from build123d import *

# Parameters (mm, degrees)
BOSS_EXTRU_1_DEPTH      = 55
ESQUISSE2_W             = 35.5
ESQUISSE2_H             = 2
BOSS_EXTRU_2_DEPTH      = 1
BOSS_EXTRU_3_DEPTH      = 31.5
ESQUISSE4_W             = 8
ESQUISSE4_H             = 6.5
BOSS_EXTRU_4_DEPTH      = 2
ESQUISSE5_W             = 4.9
ESQUISSE5_H             = 1.9
BOSS_EXTRU_5_DEPTH      = 2
BOSS_EXTRU_6_DEPTH      = 3
ESQUISSE8_W             = 29.5
ESQUISSE8_H             = 49
ENL_V_MAT_EXTRU_2_DEPTH = 1
CONG_1_R                = 2
CONG_4_R                = 1.5
ESQUISSE7_R             = 6
ENL_V_MAT_EXTRU_1_DEPTH = 67.304223093


with BuildPart() as part:
    # Esquisse1 → Boss.-Extru.1 (new body)
    with BuildSketch(Plane.XY):
        Polygon((0, 0), (-2, 0), (-2, -1), (33.5, -1), (33.5, 0), (31.5, 0), (31.5, 2), (0, 2), align=None)
    extrude(amount=BOSS_EXTRU_1_DEPTH)

    # Esquisse2 → Boss.-Extru.2 (add)
    with BuildSketch(Plane.XZ.offset(1)):
        with Locations((15.75, 56)):
            Rectangle(ESQUISSE2_W, ESQUISSE2_H)
    extrude(amount=-BOSS_EXTRU_2_DEPTH)

    # Esquisse3 → Boss.-Extru.3 (add)
    with BuildSketch(Plane.ZY):
        Polygon((55, 2), (55, 2.1), (57, 2.1), (57, 4.1), (53, 4.1), (53, 2), align=None)
    extrude(amount=-BOSS_EXTRU_3_DEPTH)

    # Esquisse4 → Boss.-Extru.4 (add)
    with BuildSketch(Plane(origin=(0, 0, 0), x_dir=(-1, 0, 0), z_dir=(0, 0, -1))):
        with Locations((-15.75, 3.75)):
            Rectangle(ESQUISSE4_W, ESQUISSE4_H)
    extrude(amount=BOSS_EXTRU_4_DEPTH)

    # Esquisse5 → Boss.-Extru.5 (add)
    with BuildSketch(Plane.XY):
        with Locations((15.75, 5)):
            Rectangle(ESQUISSE5_W, ESQUISSE5_H)
    extrude(amount=BOSS_EXTRU_5_DEPTH)

    # Esquisse6 → Boss.-Extru.6 (add)
    with BuildSketch(Plane.XZ.offset(1)):
        with BuildLine():
            Line((5.75, 0), (5.75, -5))
            ThreePointArc((5.75, -5), (7.214466094, -8.535533906), (10.75, -10))
            Line((10.75, -10), (20.75, -10))
            ThreePointArc((20.75, -10), (24.285533906, -8.535533906), (25.75, -5))
            Line((25.75, -5), (25.75, 0))
            Line((25.75, 0), (5.75, 0))
        make_face()
    extrude(amount=-BOSS_EXTRU_6_DEPTH)

    # Esquisse8 → Enlèv. mat.-Extru.2 (cut)
    with BuildSketch(Plane(origin=(0, 2, 0), x_dir=(1, 0, 0), z_dir=(0, 1, 0))):
        with Locations((15.75, -26.5)):
            Rectangle(ESQUISSE8_W, ESQUISSE8_H)
    extrude(amount=-ENL_V_MAT_EXTRU_2_DEPTH, mode=Mode.SUBTRACT)

    # Congé1
    cong_1_edges = [part.edges().sort_by_distance(p)[0] for p in [
        (15.75, 2, 53),
    ]]
    fillet(cong_1_edges, radius=CONG_1_R - 0.0001)  # a hair under: the kernel refuses the full size

    # Congé4
    cong_4_edges = [part.edges().sort_by_distance(p)[0] for p in [
        (11.75, 7, -1),
        (19.75, 7, -1),
        (15.75, 7, -2),
        (19.75, 4.5, -2),
        (11.75, 4.5, -2),
        (15.75, 2, -2),
        (11.75, 2, -1),
        (19.75, 2, -1),
    ]]
    fillet(cong_4_edges, radius=CONG_4_R)

    # Esquisse7 → Enlèv. mat.-Extru.1 (cut, through all)
    with BuildSketch(Plane(origin=(0, 2, 0), x_dir=(1, 0, 0), z_dir=(0, 1, 0))):
        with Locations(Location((15.75, -15, 0), (0, 0, 180))):
            Circle(ESQUISSE7_R)
        with Locations(Location((15.75, -40, 0), (0, 0, 180))):
            Circle(ESQUISSE7_R)
    extrude(amount=-ENL_V_MAT_EXTRU_1_DEPTH, mode=Mode.SUBTRACT)


solid = part.part
Check sheet for the modelled part. Datum: model origin and axes. Units: mm. A direction names the side the tool comes from. Coordinates: 2 decimals unless noted, no trailing zeros. Loops run counter-clockwise (first coordinate to the right, second up) from the corner with the lowest first, then second, coordinate; pieces in that order, holes last. Notation, with made-up numbers: (61.25, 75) -> (76.25, 75) arc R25 cw to (76.25, 87) -> close; hole circle Ø7 at (78.5, -21.5). An arc over 180 degrees is marked (long way). Write item = value, one per line. Start each with the question number.
1. Section check D-D on z = 41. Record the cut outline in (x, y).
2. Depth check by flat-ended pin: P1, Ø15.5, axis at x = 15.75, z = 40, coming from the +Y side; P2, Ø1.5, axis at y = 5, z = 1.5, coming from the +X side; P3, Ø0.6, axis at x = 17, y = 4.5, coming from the -Z side. Enter the tip coordinate at first touch or a pass-through.
3. Draft check along Y on faces 1 (the cylindrical face through (11.3, 2.43, -0.25)), 2 (the flat face through (16, 2.1, 56)), 3 (the cylindrical face through (24.25, 0.48, -8.57)). Enter one of: released by +Y, released by -Y, zero draft, split by the parting line, or undercut.
4. Section check A-A on x = 15.75. Give the number of separate pieces and of enclosed holes in the cut face, then the cut area to 3 significant figures.
5. Material ranges on line 1 (Z direction, x = 15.75, y = 0.35); line 2 (X direction, y = 1.5, z = 20.5); line 3 (X direction, y = 0.5, z = 26), recorded low to high.
6. Tool access check on faces 4 (the flat face through (5.75, 0, -2)), 5 (the flat face through (16, 4.1, 55)), 6 (the flat face through (-1, 0, 35)), 7 (the flat face through (16, 1, 26)), 8 (the flat face through (31.5, 1, 28)). Record the directions out of +Z, -Z, +X, -X, +Y, -Y that give a thin tool (end or side, any length) a straight path to the whole face; none if there is none.
7. Section check B-B on z = 15. Record the cut outline in (x, y).
8. Section check C-C on z = 28.5. Record the cut outline in (x, y), then the cut area to 3 significant figures.
Responses:
q1.outline = (-2, -1) -> (9.83, -1) -> (9.83, 1) -> (1, 1) -> (1, 2) -> (0, 2) -> (0, 0) -> (-2, 0) -> close; (21.67, -1) -> (33.5, -1) -> (33.5, 0) -> (31.5, 0) -> (31.5, 2) -> (30.5, 2) -> (30.5, 1) -> (21.67, 1) -> close
q2.P1 = 1
q2.P2 = 18.2
q2.P3 = -2
q3.face_1 = released by +Y
q3.face_2 = undercut
q3.face_3 = zero draft
q4.separate_pieces = 3
q4.enclosed_holes = 0
q4.area = 123 mm2
q5.line_1 = -10 to 9, 21 to 34, 46 to 55
q5.line_2 = 0 to 1, 30.5 to 31.5
q5.line_3 = 0 to 31.5
q6.face_4 = -Z, -X, +Y, -Y
q6.face_5 = +Z, +X, -X, +Y
q6.face_6 = +Z
q6.face_7 = +Y
q6.face_8 = +Z, -Z, +X, +Y
q7.outline = (-2, -1) -> (9.75, -1) -> (9.75, 1) -> (1, 1) -> (1, 2) -> (0, 2) -> (0, 0) -> (-2, 0) -> close; (21.75, -1) -> (33.5, -1) -> (33.5, 0) -> (31.5, 0) -> (31.5, 2) -> (30.5, 2) -> (30.5, 1) -> (21.75, 1) -> close
q8.outline = (-2, -1) -> (33.5, -1) -> (33.5, 0) -> (31.5, 0) -> (31.5, 2) -> (30.5, 2) -> (30.5, 1) -> (1, 1) -> (1, 2) -> (0, 2) -> (0, 0) -> (-2, 0) -> close
q8.area = 69.0 mm2
